from build123d import *

# Parameters (mm, degrees)
F1_DEPTH      = 25
F2_W          = 35
F2_H          = 10
F3_DEPTH      = 40
F5_DEPTH      = 5
F5_DEPTH_BACK = 5
F6_R          = 3
F7_DEPTH      = 25


with BuildPart() as f1:
    # F0 (on Front) → F1 (new body)
    with BuildSketch(Plane.XZ):
        Polygon((17.5, -7.2487373415), (17.5, 7.2487373415), (7.2487373415, 17.5), (-7.2487373415, 17.5), (-17.5, 7.2487373415), (-17.5, -7.2487373415), (-7.2487373415, -17.5), (7.2487373415, -17.5), align=None)
        Polygon((4.1421356237, 10), (10, 4.1421356237), (10, -4.1421356237), (4.1421356237, -10), (-4.1421356237, -10), (-10, -4.1421356237), (-10, 4.1421356237), (-4.1421356237, 10), align=None, mode=Mode.SUBTRACT)
    extrude(amount=F1_DEPTH)

    # F2 (on face) → F3 (cut)
    with BuildSketch(Plane.XZ.offset(25)):
        with Locations((0, 14.2487373415)):
            Rectangle(F2_W, F2_H)
    extrude(amount=-F3_DEPTH, mode=Mode.SUBTRACT)

    # F4 (on face) → F5 (cut, two sides)
    with BuildSketch(Plane.XY.offset(-10)) as f5_sk:
        Polygon((3.1754264805, -7), (-3.1754264805, -7), (-6.3508529611, -12.5), (-3.1754264805, -18), (3.1754264805, -18), (6.3508529611, -12.5), align=None)
    extrude(amount=-F5_DEPTH, mode=Mode.SUBTRACT)
    extrude(f5_sk.sketch, amount=F5_DEPTH_BACK, mode=Mode.SUBTRACT)

    # F6 (on face) → F7 (cut)
    with BuildSketch(Plane(origin=(0, 0, -17.5), x_dir=(1, 0, 0), z_dir=(0, 0, -1))):
        with Locations((0, 12.5)):
            Circle(F6_R)
    extrude(amount=-F7_DEPTH, mode=Mode.SUBTRACT)


solid = f1.part
Geometry check sheet. Reference: the model listing, model coordinates, mm. A direction names the side the tool comes from. Coordinates: 2 decimals unless noted, no trailing zeros. Order: outer loops, then holes, each group sorted by start corner. A loop starts at its lowest first (then second) coordinate and runs counter-clockwise, first axis right, second up. Notation, with made-up numbers: (-0.5, 85) -> (41.5, 85) arc R23 ccw to (41.5, 123) -> close; hole circle Ø8 at (-37, -37). An arc over 180 degrees is marked (long way). Use a Markdown table: item, result. Add a question column.
1. Material ranges on L1, parallel to Y at x = 0, z = -16.85; L2, parallel to X at y = -5.75, z = -2.5; L3, parallel to X at y = -4, z = 4.75, recorded low to high.
2. Cross-section at A-A (z = -2). Enter the section's corners in (x, y), and give its area (3 significant figures).
3. Mould release check, pull along Y, two halves, no side actions. Record for faces 6 (the face through (8, 0, -7)), 7 (the face through (17.5, -12, 0)), 8 (the face through (4.785, -9.788, -12.146)): pulls with the +Y half, pulls with the -Y half, needs draft (parallel to the pull), parting line crosses it, or undercut.
4. Cross-section at B-B (x = 0). Enter the section's corners in (y, z), and give its area (4 significant figures).
5. Set-up check for faces 1 (the face through (4.74, -15.29, -12.25)), 2 (the face through (0, -18, -12)), 3 (the face through (0, -3, -10)), 4 (the face through (-7.03, -12.32, -7.11)), 5 (the face through (-10, -13, 9.249)): record each of +Z, -Z, +X, -X, +Y, -Y from which the full face is reachable in a straight line by a thin tool's end or side.
6. Go/stop test with flat-tipped pins: pin 1 Ø2 at (x, y) = (-13, -9.5) entering from -Z; pin 2 Ø6.5 at (x, y) = (-0.5, -6) entering from +Z; pin 3 Ø7 at (x, y) = (0, -12.5) entering from +Z. Record where each tip stops, or that it passes through.
7. Cross-section at C-C (y = -22.75). Enter the section's corners in (x, z).
Filled sheet:
| question | item | result |
|---|---|---|
| 1 | L1 | -25 to -15.5, -9.5 to 0 |
| 1 | L2 | -17.5 to -10, 10 to 17.5 |
| 1 | L3 | -17.5 to -9.39, 9.39 to 17.5 |
| 2 | outline | (-17.5, -25) -> (-10, -25) -> (-10, 0) -> (-17.5, 0) -> close; (10, -25) -> (17.5, -25) -> (17.5, 0) -> (10, 0) -> close |
| 2 | area | 375 mm2 |
| 3 | face 6 | pulls with the +Y half |
| 3 | face 7 | needs draft |
| 3 | face 8 | undercut |
| 4 | outline | (-25, -17.5) -> (-15.5, -17.5) -> (-15.5, -15) -> (-18, -15) -> (-18, -10) -> (-25, -10) -> close; (-9.5, -17.5) -> (0, -17.5) -> (0, -10) -> (-7, -10) -> (-7, -15) -> (-9.5, -15) -> close |
| 4 | area | 117.5 mm2 |
| 5 | face 1 | none |
| 5 | face 2 | +Z |
| 5 | face 3 | +Z, +Y, -Y |
| 5 | face 4 | +Y, -Y |
| 5 | face 5 | +Z, +X, -X, +Y, -Y |
| 6 | pin 1 | z = -12.75 |
| 6 | pin 2 | z = -10 |
| 6 | pin 3 | z = -15 |
| 7 | outline | (-17.5, -7.25) -> (-7.25, -17.5) -> (7.25, -17.5) -> (17.5, -7.25) -> (17.5, 7.25) -> (15.5, 9.25) -> (4.89, 9.25) -> (10, 4.14) -> (10, -4.14) -> (4.14, -10) -> (-4.14, -10) -> (-10, -4.14) -> (-10, 4.14) -> (-4.89, 9.25) -> (-15.5, 9.25) -> (-17.5, 7.25) -> close |
